Design review of the part shown in the three views and the two pictorial views. Dimensions are in mm from the part's minimum x, y and z. A direction names the side the tool comes from. Round coordinates to 2 decimals unless told otherwise and drop trailing zeros. Write each loop counter-clockwise with the first axis right and the second up, starting at its lowest first coordinate (ties: lowest second). Pieces come first, ordered by that corner, then holes. Notation, with made-up numbers: (49, -39.75) -> (56, -39.75) arc R9 cw to (56, -27.75) -> close; hole circle Ø11 at (38, -22.5). An arc over 180 degrees is marked (long way). Answer as a JSON object with one key per item and string values. Group by question number.
1) We need section C-C, the plane y = 3.2. Write out the cut boundary in (x, z) (3 decimals).
2) Mouldability with a two-part tool opening along Y and no side actions: class the marked faces 3, 4 and 5 as pulls with the +Y half, pulls with the -Y half, needs draft (parallel to the pull), parting line crosses it, or undercut.
3) Insertion check: pin 1 Ø1.7 at (x, z) = (2.5, 3.125) entering from -Y; pin 2 Ø1.2 at (x, z) = (17.8, 3.125) entering from -Y. Each pin has a flat end and moves straight along its axis. Give the tip position at first contact, or say it passes through.
4) To check wall thickness, follow probe 1 along Z at (x, y) = (17.8, 1.85) (3 decimals); probe 2 along Y at (x, z) = (11.25, 4) (3 decimals); probe 3 along X at (y, z) = (3.9, 3.5). State the ranges of each line that lie inside material, in increasing order. Write a range as [from, to].
5) Machinability: for the marked faces 1 and 2, which of the approach directions +Z, -Z, +X, -X, +Y, -Y give a long, thin tool a straight path to every point of the face, cutting with its end or side? Answer none if there is none.
6) We need section D-D, the plane x = 9. Write out the cut boundary in (y, z) (3 decimals).
7) We need section B-B, the plane z = 4.25. Write out the cut boundary in (x, y) (3 decimals).
8) We need section A-A, the plane x = 17.8. Write out the cut boundary in (y, z) (3 decimals).
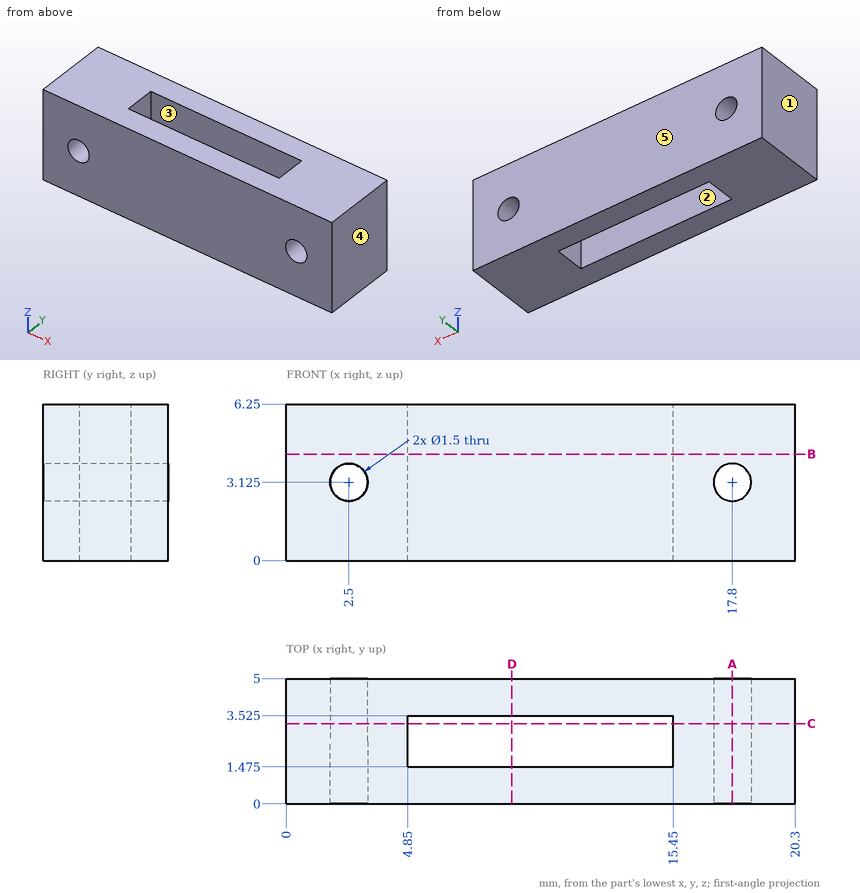
Here are the results:
{
 "1": {"outline": "(0, 0) -> (4.85, 0) -> (4.85, 6.25) -> (0, 6.25) -> close; (15.45, 0) -> (20.3, 0) -> (20.3, 6.25) -> (15.45, 6.25) -> close; hole circle Ø1.5 at (2.5, 3.125); hole circle Ø1.5 at (17.8, 3.125)"},
 "2": {"face 3": "undercut", "face 4": "needs draft", "face 5": "pulls with the +Y half"},
 "3": {"pin 1": "stops at y = 0", "pin 2": "passes through"},
 "4": {"probe 1": "z = [0, 2.375], [3.875, 6.25]", "probe 2": "y = [0, 1.475], [3.525, 5]", "probe 3": "x = [0, 1.85], [3.15, 17.15], [18.45, 20.3]"},
 "5": {"face 1": "+Z, -Z, -X, +Y, -Y", "face 2": "+Z, -Z"},
 "6": {"outline": "(0, 0) -> (1.475, 0) -> (1.475, 6.25) -> (0, 6.25) -> close; (3.525, 0) -> (5, 0) -> (5, 6.25) -> (3.525, 6.25) -> close"},
 "7": {"outline": "(0, 0) -> (20.3, 0) -> (20.3, 5) -> (0, 5) -> close; hole (4.85, 1.475) -> (15.45, 1.475) -> (15.45, 3.525) -> (4.85, 3.525) -> close"},
 "8": {"outline": "(0, 0) -> (5, 0) -> (5, 2.375) -> (0, 2.375) -> close; (0, 3.875) -> (5, 3.875) -> (5, 6.25) -> (0, 6.25) -> close"}
}
